Read the model definition and answer for the solid it produces. Units are mm, in the model's axes. A direction names the side the tool comes from. Round coordinates to 2 decimals unless told otherwise and drop trailing zeros. Order: outer loops, then holes, each group sorted by start corner. A loop starts at its lowest first (then second) coordinate and runs counter-clockwise, first axis right, second up. Notation, with made-up numbers: (-20.75, 88) - (18.25, 88) arc R30 ccw to (18.25, 119) - close; hole circle Ø8 at (23, 35). An arc over 180 degrees is marked (long way). Answer as a JSON object with one key per item and string values. Group by question number.
Q1. A cutting plane is placed at C-C on z = -32. Determine the outline of the cut face in (x, y), and give its area (3 significant figures).
Q2. A tool of negligible diameter and unlimited length cuts with its end or side. For faces 1 (the cylindrical face through (5.723, -1.802, -308.056)), 2 (the flat face through (0, 0, -1.5)), 3 (the cylindrical face through (5.723, -1.802, -19.07)), from which of +Z, -Z, +X, -X, +Y, -Y can it reach the whole face along a straight path? Write none if from no direction.
Q3. A cutting plane is placed at A-A on y = 0. Determine the outline of the cut face in (x, z).
Q4. Consider line 1 (X direction, y = 0.25, z = -149); line 2 (Z direction, x = -0.25, y = -3.75); line 3 (Z direction, x = 2, y = 5.75). Determine where each line is inside the solid, lowest interval first.
Q5. Given pin 1 Ø5 at (x, z) = (-4, -209.5) entering from -Y; pin 2 Ø6 at (x, y) = (6.5, 0) entering from +Z; pin 3 Ø1.5 at (y, z) = (3.5, -53) entering from +X; pin 4 Ø6 at (x, y) = (-2.5, 3.5) entering from +Z, each flat-ended and moving along its own axis, determine where each tip first touches the part or whether it passes through.
```python
from build123d import *


with BuildPart() as part:
    # Schizzo2 → Rivoluzione2 (revolve)
    with BuildSketch(Plane(origin=(0, 0, 0), x_dir=(0, 0, -1), z_dir=(1, 0, 0)), mode=Mode.PRIVATE) as rivoluzione2_sk:
        Polygon((1.5, 0), (1.5, 3), (8.5, 3), (8.5, 4), (14, 4), (14, 6), (24, 6), (24, 8), (304, 8), (304, 6), (312, 6), (312, 4), (331, 4), (331, 0), align=None)
    revolve(rivoluzione2_sk.sketch.rotate(Axis((0, 0, 0), (0, 0, -1)), 90), axis=Axis((0, 0, 0), (0, 0, -1)))


solid = part.part
```
Result set:
{
 "1": {"outline": "circle Ø16 at (0, 0)", "area": "201 mm²"},
 "2": {"face 1": "-Z", "face 2": "+Z, +X, -X, +Y, -Y", "face 3": "+Z"},
 "3": {"outline": "(-8, -304) - (-6, -304) - (-6, -312) - (-4, -312) - (-4, -331) - (4, -331) - (4, -312) - (6, -312) - (6, -304) - (8, -304) - (8, -24) - (6, -24) - (6, -14) - (4, -14) - (4, -8.5) - (3, -8.5) - (3, -1.5) - (-3, -1.5) - (-3, -8.5) - (-4, -8.5) - (-4, -14) - (-6, -14) - (-6, -24) - (-8, -24) - close"},
 "4": {"line 1": "x = -8 to 8", "line 2": "z = -331 to -8.5", "line 3": "z = -304 to -24"},
 "5": {"pin 1": "stops at y = -7.86", "pin 2": "stops at z = -8.5", "pin 3": "stops at x = 7.51", "pin 4": "stops at z = -1.5"}
}
